For this review, take the finished solid that the model builds, in its own axes (mm). Give positions to 0.01 mm unless a question says otherwise; leave off trailing zeros. Loops run counter-clockwise (first coordinate to the right, second up) from the corner with the lowest first, then second, coordinate; pieces in that order, holes last.
```python
from build123d import *

# Parameters (mm, degrees)
F1_DEPTH = 406.35
F2_W     = 7.94
F2_H     = 6.35
F3_DEPTH = 1200.001


with BuildPart() as f1:
    # F0 (on Front) → F1 (new body)
    with BuildSketch(Plane.XZ):
        Polygon((-29.519806, 967.791521), (-45.394806, 967.791521), (-45.394806, -232.208479), (-29.519806, -232.208479), (-29.519806, 95.731521), (-37.459806, 95.731521), (-37.459806, 111.606521), (-29.519806, 111.606521), (-29.519806, 431.606521), (-37.459806, 431.606521), (-37.459806, 447.481521), (-29.519806, 447.481521), (-29.519806, 695.731521), (-37.459806, 695.731521), (-37.459806, 711.606521), (-29.519806, 711.606521), align=None)
    extrude(amount=F1_DEPTH)

    # F2 (on face) → F3 (cut, through all)
    with BuildSketch(Plane.XY.offset(967.791521)):
        with Locations((-33.489806, -3.175)):
            Rectangle(F2_W, F2_H)
    extrude(amount=-F3_DEPTH, mode=Mode.SUBTRACT)


solid = f1.part
```
Q1. For pin 1 Ø2.5 at (x, z) = (-32.5, 797.5) entering from +Y, flat-tipped, find the tip position at first contact; note if it passes through.
Answers:
pin 1: stops at y = -6.35
Q2. Mouldability with a two-part tool opening along Z and no side actions: class faces 1 (the flat face through (-29.52, -204, 269)), 2 (the flat face through (-37.46, -204, 104)) as +Z half, -Z half, draft (parallel to the pull), parting line (faces both ways), or undercut.
Answers:
face 1: draft
face 2: undercut
Q3. Consider section A-A on y = -211.5. Give the boundary of the cut face in (x, z).
Answers:
outline: (-45.39, -232.21) - (-29.52, -232.21) - (-29.52, 95.73) - (-37.46, 95.73) - (-37.46, 111.61) - (-29.52, 111.61) - (-29.52, 431.61) - (-37.46, 431.61) - (-37.46, 447.48) - (-29.52, 447.48) - (-29.52, 695.73) - (-37.46, 695.73) - (-37.46, 711.61) - (-29.52, 711.61) - (-29.52, 967.79) - (-45.39, 967.79) - close
Q4. For probe 1 along Z at (x, y) = (-32.75, -386.5); probe 2 along Y at (x, z) = (-34.5, 841); probe 3 along X at (y, z) = (-96, 438), list the stretches that pass through material, from the lowest coordinate up.
Answers:
probe 1: z = -232.21 to 95.73, 111.61 to 431.61, 447.48 to 695.73, 711.61 to 967.79
probe 2: y = -406.35 to -6.35
probe 3: x = -45.39 to -37.46
